```python
from build123d import *

# Parameters (mm, degrees)
SKETCH1_R           = 1.6
SKETCH1_W           = 6
SKETCH1_H           = 3
BOSS_EXTRUDE1_DEPTH = 2
FILLET1_R           = 1
SKETCH3_R           = 0.5
CUT_EXTRUDE1_DEPTH  = 2
SKETCH4_W           = 8.927318102
SKETCH4_H           = 47.063450143
SKETCH4_W_2         = 9.73496377
SKETCH4_H_2         = 34.688645835
CUT_EXTRUDE2_DEPTH  = 2
EXTRUDE_THIN1_DEPTH = 2
FILLET2_R           = 1.5


with BuildPart() as part:
    # Sketch1 → Boss-Extrude1 (new body)
    # profile 1 of 5: a face of its own
    with BuildSketch(Plane(origin=(0, 0, 0), x_dir=(1, 0, 0), z_dir=(0, 1, 0))):
        Polygon((6, 10), (0, 10), (-5, 10), (-5, -57.026436391), (0, -57.026436391), (6, -57.026436391), (10.662281872, -57.026436391), (16.662281872, -57.026436391), (21.662281872, -57.026436391), (21.662281872, 10), (16.662281872, 10), (10.662281872, 10), align=None)
        with Locations(Location((16.662281872, -47.026436391, 0), (0, 0, 270))):
            Circle(SKETCH1_R, mode=Mode.SUBTRACT)
        with Locations(Location((0, 0, 0), (0, 0, 270))):
            Circle(SKETCH1_R, mode=Mode.SUBTRACT)
        with Locations(Location((16.662281872, 0, 0), (0, 0, 270))):
            Circle(SKETCH1_R, mode=Mode.SUBTRACT)
    # profile 2 of 5: a face of its own
    with BuildSketch(Plane(origin=(0, 0, 0), x_dir=(1, 0, 0), z_dir=(0, 1, 0))):
        with Locations((13.662281872, 11.5)):
            Rectangle(SKETCH1_W, SKETCH1_H)
    # profile 3 of 5: a face of its own
    with BuildSketch(Plane(origin=(0, 0, 0), x_dir=(1, 0, 0), z_dir=(0, 1, 0))):
        with Locations((3, 11.5)):
            Rectangle(SKETCH1_W, SKETCH1_H)
    # profile 4 of 5: a face of its own
    with BuildSketch(Plane(origin=(0, 0, 0), x_dir=(1, 0, 0), z_dir=(0, 1, 0))):
        with Locations((3, -58.526436391)):
            Rectangle(SKETCH1_W, SKETCH1_H)
    # profile 5 of 5: a face of its own
    with BuildSketch(Plane(origin=(0, 0, 0), x_dir=(1, 0, 0), z_dir=(0, 1, 0))):
        with Locations((13.662281872, -58.526436391)):
            Rectangle(SKETCH1_W, SKETCH1_H)
    extrude(amount=BOSS_EXTRUDE1_DEPTH)

    # Fillet1
    fillet1_edges = [part.edges().sort_by_distance(p)[0] for p in [
        (21.662281872, 1, 57.026436391),
        (16.662281872, 1, 60.026436391),
        (10.662281872, 1, 60.026436391),
        (6, 1, 60.026436391),
        (0, 1, 60.026436391),
        (-5, 1, 57.026436391),
        (-5, 1, -10),
        (0, 1, -13),
        (6, 1, -13),
        (10.662281872, 1, -13),
        (16.662281872, 1, -13),
        (21.662281872, 1, -10),
    ]]
    fillet(fillet1_edges, radius=FILLET1_R)

    # Sketch3 → Cut-Extrude1 (cut)
    with BuildSketch(Plane.XZ):
        with Locations((0, 57.026436391)):
            Circle(SKETCH3_R)
        with Locations((6, 57.026436391)):
            Circle(SKETCH3_R)
        with Locations((10.662281872, 57.026436391)):
            Circle(SKETCH3_R)
        with Locations((16.662281872, 57.026436391)):
            Circle(SKETCH3_R)
        with Locations((0, -10)):
            Circle(SKETCH3_R)
        with Locations((6, -10)):
            Circle(SKETCH3_R)
        with Locations((10.662281872, -10)):
            Circle(SKETCH3_R)
        with Locations((16.662281872, -10)):
            Circle(SKETCH3_R)
    extrude(amount=-CUT_EXTRUDE1_DEPTH, mode=Mode.SUBTRACT)

    # Sketch4 → Cut-Extrude2 (cut)
    with BuildSketch(Plane(origin=(0, 2, 0), x_dir=(1, 0, 0), z_dir=(0, 1, 0))):
        with Locations((3.463659051, -28.49471132)):
            Rectangle(SKETCH4_W, SKETCH4_H)
        with Locations((12.794799987, -22.307309166)):
            Rectangle(SKETCH4_W_2, SKETCH4_H_2)
        Polygon((7.927318102, -39.651632083), (7.927318102, -46.759423391), (17.662281872, -39.651632083), align=None)
    extrude(amount=-CUT_EXTRUDE2_DEPTH, mode=Mode.SUBTRACT)

    # Sketch6 → Extrude-Thin1 (add)
    with BuildSketch(Plane(origin=(0, 2, 0), x_dir=(1, 0, 0), z_dir=(0, 1, 0))):
        Polygon((-2.318677564, -5.677891475), (17.181124518, -41.646227603), (19.818479645, -40.216417149), (0.318677564, -4.248081021), align=None)
        Polygon((16.267906789, -4.410068416), (-2.394375083, -51.473518559), (0.394375083, -52.579354223), (19.056656955, -5.51590408), align=None)
    extrude(amount=-EXTRUDE_THIN1_DEPTH)

    # Fillet2
    fillet2_edges = [part.edges().sort_by_distance(p)[0] for p in [
        (7.927318102, 1, 46.759423391),
        (7.927318102, 1, 52.026436391),
        (17.662281872, 1, 9.032306985),
        (17.662281872, 1, 36.239205179),
        (16.048655791, 1, 4.962986248),
        (0.706254859, 1, 4.962986248),
        (-1, 1, 47.957115655),
        (-1, 1, 8.110256565),
        (0.613626081, 1, 52.026436391),
        (16.542874861, 1, 40.468944978),
        (9.989723555, 1, 28.381337735),
        (9.567384345, 1, 21.307771825),
        (11.431310298, 1, 24.745874168),
        (8.125797601, 1, 24.943235392),
    ]]
    fillet(fillet2_edges, radius=FILLET2_R)


solid = part.part
```
Geometry check sheet. Reference: the model listing, model coordinates, mm. A direction names the side the tool comes from. Give positions to 0.01 mm unless a question says otherwise; leave off trailing zeros. Write each loop counter-clockwise with the first axis right and the second up, starting at its lowest first coordinate (ties: lowest second). Pieces come first, ordered by that corner, then holes.
1) Section check A-A, the plane z = 0. Record the boundary of the cut face in (x, y).
2) Section check B-B, the plane z = 11. Record the boundary of the cut face in (x, y).
3) Gauge pin test, flat ends, axial feed: pin 1 (0.8 mm diameter, centred on y = 0.5, z = -11.5, fed in from +X); pin 2 (0.8 mm diameter, centred on y = 1, z = -11.5, fed in from -X); pin 3 (0.6 mm diameter, centred on x = -3, y = 1, fed in from -Z). Record the tip position at first contact, or that the pin passes through.
4) Access from +Z, -Z, +X, -X, +Y, -Y to the whole of each face (thin tool, end or side, straight path). Record for faces 1 (the flat face through (-2, 1, 57.026)), 2 (the flat face through (8, 1, 57.026)), 3 (the cylindrical face through (9.42, 0.99, 19.27)).
5) Section check C-C, the plane x = 4.25. Record the boundary of the cut face in (y, z).
6) Release check for a two-part mould opening along X. For faces 4 (the flat face through (16.662, 1, 58)), 5 (the cylindrical face through (16.472, 0.986, 15.417)), 6 (the cylindrical face through (15.069, 1.014, 5.603)), 7 (the flat face through (3, 1, -13)) record: pulls with the +X half, pulls with the -X half, needs draft (parallel to the pull), parting line crosses it, or undercut.
7) Material ranges on L1, parallel to X at y = 1.4, z = 0; L2, parallel to X at y = 1.7, z = 23.5; L3, parallel to Z at x = 9.75, y = 0.75, recorded low to high.
8) Section check D-D, the plane y = 0.85. State how many separate pieces and enclosed holes the cut face has, and give its area (3 significant figures).
Computed:
1. outline: (-5, 0) - (-1.6, 0) - (-1.6, 2) - (-5, 2) - close; (1.6, 0) - (15.06, 0) - (15.06, 2) - (1.6, 2) - close; (18.26, 0) - (21.66, 0) - (21.66, 2) - (18.26, 2) - close
2. outline: (-5, 0) - (3.98, 0) - (3.98, 2) - (-5, 2) - close; (13.65, 0) - (21.66, 0) - (21.66, 2) - (13.65, 2) - close
3. pin 1: stops at x = 16.66
3. pin 2: stops at x = 0
3. pin 3: stops at z = -10
4. face 1: +Z, -X, +Y, -Y
4. face 2: +Z, +Y, -Y
4. face 3: +Y, -Y
5. outline: (0, -13) - (2, -13) - (2, 4.96) - (0, 4.96) - close; (0, 11.5) - (2, 11.5) - (2, 17.79) - (0, 17.79) - close; (0, 34.72) - (2, 34.72) - (2, 42.86) - (0, 42.86) - close; (0, 52.03) - (2, 52.03) - (2, 60.03) - (0, 60.03) - close
6. face 4: pulls with the +X half
6. face 5: undercut
6. face 6: undercut
6. face 7: needs draft
7. L1: x = -5 to -1.6, 1.6 to 15.06, 18.26 to 21.66
7. L2: x = -5 to -1, 7.34 to 11.93, 17.66 to 21.66
7. L3: z = -10 to 4.96, 19.22 to 30.49, 45.43 to 57.03
8. separate pieces: 1
8. enclosed holes: 7
8. area: 1,320 mm2
